```python
from build123d import *

# Parameters (mm, degrees)
F1_DEPTH  = 10
F2_R      = 4
F3_DEPTH  = 25
F7_DEPTH  = 25
F8_R      = 4
F9_DEPTH  = 5
F10_DEPTH = 5


# Not quite as in the source:
# - after a boolean that leaves OpenCascade's solid faulty, fix() repairs it


with BuildPart() as f1:
    # F0 (on Top) → F1 (new body)
    with BuildSketch(Plane.XY):
        Polygon((0, 0), (86.6025403784, 50), (71.6025403784, 50), (0, 50), align=None)
        Polygon((-86.6025403784, 50), (0, 0), (0, 50), (-71.6025403784, 50), align=None)
        Polygon((0, 120), (15, 120), (15, 150), (-15, 150), (-15, 120), align=None)
        Polygon((10, 125), (0, 125), (-10, 125), (-10, 127.5), (-10, 145), (10, 145), (10, 127.5), align=None, mode=Mode.SUBTRACT)
        with BuildLine():
            Line((71.6025403784, 50), (86.6025403784, 50))
            Line((86.6025403784, 50), (48.027253047, 87.7119317126))
            ThreePointArc((48.027253047, 87.7119317126), (35.9639012974, 93.309151767), (23.2645159855, 97.2561684211))
            Line((23.2645159855, 97.2561684211), (71.6025403784, 50))
        make_face()
        with BuildLine():
            Line((-48.027253047, 87.7119317126), (-86.6025403784, 50))
            Line((-86.6025403784, 50), (-71.6025403784, 50))
            Line((-71.6025403784, 50), (-23.2645159855, 97.2561684211))
            ThreePointArc((-23.2645159855, 97.2561684211), (-35.9639012974, 93.309151767), (-48.027253047, 87.7119317126))
        make_face()
        with BuildLine():
            ThreePointArc((23.2645159855, 97.2561684211), (35.9639012974, 93.309151767), (48.027253047, 87.7119317126))
            Line((48.027253047, 87.7119317126), (15, 120))
            Line((15, 120), (0, 120))
            Line((0, 120), (23.2645159855, 97.2561684211))
        make_face()
        with BuildLine():
            Line((-23.2645159855, 97.2561684211), (0, 120))
            Line((0, 120), (-15, 120))
            Line((-15, 120), (-48.027253047, 87.7119317126))
            ThreePointArc((-48.027253047, 87.7119317126), (-35.9639012974, 93.309151767), (-23.2645159855, 97.2561684211))
        make_face()
        Polygon((-7.5, 127.5), (7.5, 127.5), (0, 135), align=None)
        Polygon((0, 135), (7.5, 127.5), (7.5, 142.5), align=None)
        Polygon((-7.5, 142.5), (-7.5, 127.5), (0, 135), align=None)
        Polygon((0, 135), (7.5, 142.5), (-7.5, 142.5), align=None)
        Polygon((-10, 125), (0, 125), (10, 125), (10, 127.5), (7.5, 127.5), (-7.5, 127.5), (-10, 127.5), align=None)
    extrude(amount=F1_DEPTH)

    # F2 (on face) → F3 (cut)
    with BuildSketch(Plane.XY.offset(10)):
        with Locations((0, 135)):
            Circle(F2_R)
    extrude(amount=-F3_DEPTH, mode=Mode.SUBTRACT)


with BuildPart() as f4_1:
    # F4: instance of F1
    add(f1.part.mirror(Plane(origin=(-43.3012701892, 25, 5), x_dir=(0.8660254038, -0.5, 0), z_dir=(-0.5, -0.8660254038, 0))))


with BuildPart() as f1_1:
    add(f1.part)

    add(f4_1.part)  # F5 merges F4_1
    # F5: F1 across face
    add(f1.part.mirror(Plane(origin=(43.3012701892, 25, 5), x_dir=(0.8660254038, 0.5, 0), z_dir=(0.5, -0.8660254038, 0))))

    # F6 (on face) → F7 (cut)
    with BuildSketch(Plane.XY.offset(10)):
        Polygon((67.8525403784, 39.1746824527), (-67.8525403784, 39.1746824527), (0, -78.3493649054), align=None)
    extrude(amount=-F7_DEPTH, mode=Mode.SUBTRACT)

    # F8 (on face) → F9 (join)
    with BuildSketch(Plane.XY.offset(10)):
        with BuildLine():
            Line((0, 120), (-15, 120))
            Line((-15, 120), (-48.027253047, 87.7119317126))
            ThreePointArc((-48.027253047, 87.7119317126), (-35.9639012974, 93.3091517669), (-23.2645159855, 97.2561684211))
            Line((-23.2645159855, 97.2561684211), (0, 120))
        make_face()
        with BuildLine():
            Line((15, 120), (0, 120))
            Line((0, 120), (23.2645159855, 97.2561684211))
            ThreePointArc((23.2645159855, 97.2561684211), (35.9639012974, 93.3091517669), (48.027253047, 87.7119317126))
            Line((48.027253047, 87.7119317126), (15, 120))
        make_face()
        Polygon((15, 150), (-15, 150), (-15, 120), (0, 120), (15, 120), align=None)
        with Locations((0, 135)):
            Circle(F8_R, mode=Mode.SUBTRACT)
        Polygon((-7.5, 127.5), (-10, 127.5), (-10, 145), (10, 145), (10, 127.5), (7.5, 127.5), (7.5, 142.5), (-7.5, 142.5), align=None, mode=Mode.SUBTRACT)
        Polygon((137.4038105677, -62.0096189432), (111.4230484541, -47.0096189432), (103.9230484541, -60), (96.4230484541, -72.9903810568), (122.4038105677, -87.9903810568), align=None)
        Polygon((119.6586200393, -77.7451905284), (127.1586200393, -64.7548094716), (114.1682389825, -57.2548094716), (115.4182389825, -55.0897459622), (130.5736835487, -63.8397459622), (120.5736835487, -81.1602540378), (105.4182389825, -72.4102540378), (106.6682389825, -70.2451905284), align=None, mode=Mode.SUBTRACT)
        with Locations((116.9134295109, -67.5)):
            Circle(F8_R, mode=Mode.SUBTRACT)
        with BuildLine():
            Line((111.4230484541, -47.0096189432), (99.9743876016, -2.2631446437))
            ThreePointArc((99.9743876016, -2.2631446437), (98.7900464845, -15.5089237407), (95.8585705202, -28.4804223604))
            Line((95.8585705202, -28.4804223604), (103.9230484541, -60))
            Line((103.9230484541, -60), (111.4230484541, -47.0096189432))
        make_face()
        with BuildLine():
            Line((103.9230484541, -60), (72.5940545347, -68.7757460608))
            ThreePointArc((72.5940545347, -68.7757460608), (62.826145187, -77.8002280263), (51.9471345547, -85.448787069))
            Line((51.9471345547, -85.448787069), (96.4230484541, -72.9903810568))
            Line((96.4230484541, -72.9903810568), (103.9230484541, -60))
        make_face()
        Polygon((-103.9230484541, -60), (-111.4230484541, -47.0096189432), (-137.4038105677, -62.0096189432), (-122.4038105677, -87.9903810568), (-96.4230484541, -72.9903810568), align=None)
        Polygon((-120.5736835487, -81.1602540378), (-130.5736835487, -63.8397459622), (-115.4182389825, -55.0897459622), (-114.1682389825, -57.2548094716), (-127.1586200393, -64.7548094716), (-119.6586200393, -77.7451905284), (-106.6682389825, -70.2451905284), (-105.4182389825, -72.4102540378), align=None, mode=Mode.SUBTRACT)
        with Locations((-116.9134295109, -67.5)):
            Circle(F8_R, mode=Mode.SUBTRACT)
        with BuildLine():
            ThreePointArc((-95.8585705202, -28.4804223604), (-98.7900464845, -15.5089237407), (-99.9743876016, -2.2631446437))
            Line((-99.9743876016, -2.2631446437), (-111.4230484541, -47.0096189432))
            Line((-111.4230484541, -47.0096189432), (-103.9230484541, -60))
            Line((-103.9230484541, -60), (-95.8585705202, -28.4804223604))
        make_face()
        with BuildLine():
            Line((-72.5940545347, -68.7757460608), (-103.9230484541, -60))
            Line((-103.9230484541, -60), (-96.4230484541, -72.9903810568))
            Line((-96.4230484541, -72.9903810568), (-51.9471345547, -85.448787069))
            ThreePointArc((-51.9471345547, -85.448787069), (-62.826145187, -77.8002280263), (-72.5940545347, -68.7757460608))
        make_face()
    extrude(amount=F9_DEPTH)

    # F10 (add): a face of the model
    f10_faces = [f1_1.faces().sort_by_distance(p)[0] for p in [
        (25.2159598464, -90.0197712228, 10),
    ]]
    extrude(f10_faces, amount=F10_DEPTH)

    add(f1_1.part.fix(), mode=Mode.REPLACE)


solid = f1_1.part
```
Here's how the part is built. I have some questions about the finished solid (model axes, mm). A direction names the side the tool comes from. Give positions to 0.01 mm unless a question says otherwise; leave off trailing zeros. Loops run counter-clockwise (first coordinate to the right, second up) from the corner with the lowest first, then second, coordinate; pieces in that order, holes last. Notation, with made-up numbers: (59, 12) -> (80, 12) arc R27 cw to (80, 37) -> close; hole circle Ø10 at (44.5, 15). An arc over 180 degrees is marked (long way). Use one line per item in the form item = value. Start each with the question number.
1) Imagine slicing it at B-B (x = 30.5). Please give me the cut outline in (y, z), then the cut area to 3 significant figures.
2) Imagine slicing it at C-C (y = -11). Please give me the cut outline in (x, z).
3) For P1, Ø2.5, axis at y = 134.5, z = 11.5, coming from the +X side; P2, Ø4.5, axis at y = 130.5, z = 8, coming from the -X side; P3, Ø8, axis at y = 50.5, z = 10, coming from the -X side, each with a flat end and sliding along its axis, tell me the tip position at first contact or that it passes through.
4) Which directions (+Z, -Z, +X, -X, +Y, -Y) give clear straight access to the entire face, cutting with the end or side of a thin tool? Please do faces 4 (the face through (43.802, -24.132, 7.395)), 5 (the face through (0, 150, 7)), 6 (the face through (-15, 135, 7)), 7 (the face through (15, 135, 7)).
5) Thinking about a two-plate mould opening in Y: for faces 1 (the face through (-34.401, -18.765, 7.395)), 2 (the face through (-42, -12, 15)), 3 (the face through (51.3, 84.51, 7.4)), which applies, +Y half, -Y half, draft (parallel to the pull), parting line (faces both ways), or undercut?
6) Imagine slicing it at A-A (y = 135). Please give me the cut outline in (x, z), then the cut area to 3 significant figures.
7) Please list where these lines run through material, in increasing order: line 1 along Y through (x, z) = (32, 5.25); line 2 along Y through (x, z) = (-51.5, 11.75); line 3 along X through (y, z) = (-37.5, 9.5).
Check values:
q1.outline = (-91.46, 0) -> (-80.57, 0) -> (-80.57, 15) -> (-91.46, 15) -> close; (-47.17, 0) -> (-25.52, 0) -> (-25.52, 15) -> (-47.17, 15) -> close; (39.17, 0) -> (50, 0) -> (50, 15) -> (39.17, 15) -> close; (90.18, 0) -> (104.85, 0) -> (104.85, 15) -> (90.18, 15) -> close
q1.area = 870 mm^2
q2.outline = (-102.21, 0) -> (-91.39, 0) -> (-91.39, 15) -> (-102.21, 15) -> close; (-51.38, 0) -> (-38.88, 0) -> (-38.88, 15) -> (-51.38, 15) -> close; (38.88, 0) -> (51.38, 0) -> (51.38, 15) -> (38.88, 15) -> close; (91.39, 0) -> (102.21, 0) -> (102.21, 15) -> (91.39, 15) -> close
q3.P1 = 15
q3.P2 = -15
q3.P3 = -87.5
q4.face_4 = +Z, -Z
q4.face_5 = +Z, -Z, +X, -X, +Y
q4.face_6 = +Z, -Z, -X, +Y
q4.face_7 = +Z, -Z, +X, +Y
q5.face_1 = undercut
q5.face_2 = draft
q5.face_3 = +Y half
q6.outline = (-15, 0) -> (-10, 0) -> (-10, 15) -> (-15, 15) -> close; (-7.5, 0) -> (-4, 0) -> (-4, 15) -> (-7.5, 15) -> close; (4, 0) -> (7.5, 0) -> (7.5, 15) -> (4, 15) -> close; (10, 0) -> (15, 0) -> (15, 15) -> (10, 15) -> close
q6.area = 255 mm^2
q7.line_1 = -91.04 to -80.15, -44.57 to -22.92, 39.17 to 50, 88.72 to 103.38
q7.line_2 = -85.57 to -74.68, -10.8 to 10.85, 39.17 to 50, 69.65 to 84.32
q7.line_3 = -108.99 to -98.17, -36.08 to -23.58, 23.58 to 36.08, 98.17 to 108.99
